Here's how the part is built. I have some questions about the finished solid (model axes, mm). A direction names the side the tool comes from. Coordinates: 2 decimals unless noted, no trailing zeros. Use a Markdown table: item, result. Add a question column.
Item 1: On a 3-axis mill with a long thin cutter (end or side, diameter ignored), from which of +Z, -Z, +X, -X, +Y, -Y can I reach the whole of each face in a straight line? I mean faces 5 (the flat face through (60, -156, 18.2)), 6 (the flat face through (43.6, -167, 1)), 7 (the flat face through (-43.6, -167, 1)). Say none if no direction works.
Item 2: Will these pins go through, and if not, where does the flat tip stop? pin 1 Ø2.5 at (y, z) = (-168, 2) entering from -X; pin 2 Ø4 at (y, z) = (-163, 25) entering from -X; pin 3 Ø8 at (x, y) = (6, -167) entering from +Z; pin 4 Ø1 at (x, z) = (28, 8) entering from -Y.
Item 3: If I drill on line 1 along Y through (x, z) = (26, 23); line 2 along X through (y, z) = (-155.25, 15.75); line 3 along Z through (x, y) = (-3.5, -165.5), over which ranges is the centre line in solid material (lowest first)? Write a range as from..to.
Item 4: If we mould it in two halves opening along Y, with no side actions, what happens to faces 1 (the flat face through (-53.8, -154, 17)), 2 (the cylindrical face through (-0.84, -150.65, 2)), 3 (the flat face through (-1, -155.949, 17)), 4 (the flat face through (-60, -156, 28.4))? For each: pulls with the +Y half, pulls with the -Y half, needs draft (parallel to the pull), parting line crosses it, or undercut.
```python
from build123d import *

# Parameters (mm, degrees)
EXTRUDE1_DEPTH     = 3
SKETCH3_W          = 134.4
SKETCH3_H          = 13.4
EXTRUDE2_DEPTH     = 7.4
SKETCH4_W          = 134.4
SKETCH4_H          = 13.4
SKETCH4_W_2        = 107.6
SKETCH4_H_2        = 4.4
EXTRUDE3_DEPTH     = 13
FILLET1_R          = 7
CUT_EXTRUDE1_DEPTH = 3
FILLET2_R          = 1.5
SKETCH7_R          = 2.5
EXTRUDE4_DEPTH     = 5
EXTRUDE4_TAPER     = 4
SKETCH8_R          = 2.6
CUT_EXTRUDE2_DEPTH = 5.2
CUT_EXTRUDE2_DRAFT = -3.8


with BuildPart() as part:
    # Sketch1 → Extrude1 (new body)
    with BuildSketch(Plane.XY):
        Polygon((-43.6, -161.948648405), (-43.6, -171.948648405), (43.6, -171.948648405), (43.6, -161.948648405), (67.2, -161.948648405), (67.2, -148.548648405), (-67.2, -148.548648405), (-67.2, -161.948648405), align=None)
    extrude(amount=EXTRUDE1_DEPTH)

    # Sketch3 → Extrude2 (add)
    with BuildSketch(Plane.XY.offset(3)):
        with Locations((0, -155.248648405)):
            Rectangle(SKETCH3_W, SKETCH3_H)
    extrude(amount=EXTRUDE2_DEPTH)

    # Sketch4 → Extrude3 (add)
    with BuildSketch(Plane.XY.offset(10.4)):
        with Locations((0, -155.248648405)):
            Rectangle(SKETCH4_W, SKETCH4_H)
        with Locations((0, -153.748648405)):
            Rectangle(SKETCH4_W_2, SKETCH4_H_2, mode=Mode.SUBTRACT)
    extrude(amount=EXTRUDE3_DEPTH)

    # Fillet1
    fillet1_edges = [part.edges().sort_by_distance(p)[0] for p in [
        (-67.2, -148.548648405, 11.7),
        (67.2, -148.548648405, 11.7),
        (-67.2, -155.248648405, 0),
        (0, -148.548648405, 0),
        (67.2, -155.248648405, 0),
    ]]
    fillet(fillet1_edges, radius=FILLET1_R)

    # Sketch6 → Cut-Extrude1 (cut)
    with BuildSketch(Plane.XZ.offset(161.948648405)):
        with BuildLine():
            Line((-55.3, 23.4), (-55.3, 18.9))
            ThreePointArc((-55.3, 18.9), (-53.249747468, 13.950252532), (-48.3, 11.9))
            Line((-48.3, 11.9), (48.3, 11.9))
            ThreePointArc((48.3, 11.9), (53.249747468, 13.950252532), (55.3, 18.9))
            Line((55.3, 18.9), (55.3, 23.4))
            Line((55.3, 23.4), (-55.3, 23.4))
        make_face()
    extrude(amount=-CUT_EXTRUDE1_DEPTH, mode=Mode.SUBTRACT)

    # Fillet2
    fillet2_edges = [part.edges().sort_by_distance(p)[0] for p in [
        (55.3, -158.948648405, 21.15),
        (53.249747468, -158.948648405, 13.950252532),
        (0, -158.948648405, 11.9),
        (-53.249747468, -158.948648405, 13.950252532),
        (-55.3, -158.948648405, 21.15),
        (-55.3, -161.948648405, 21.15),
        (-53.249747468, -161.948648405, 13.950252532),
        (55.3, -161.948648405, 21.15),
        (53.249747468, -161.948648405, 13.950252532),
        (0, -161.948648405, 11.9),
    ]]
    fillet(fillet2_edges, radius=FILLET2_R - 0.0001)  # a hair under: the kernel refuses the full size

    # Sketch7 → Extrude4 (add)
    with BuildSketch(Plane.XY.offset(23.4)):
        with Locations((-60.2, -155.548648405)):
            Circle(SKETCH7_R)
    extrude(amount=EXTRUDE4_DEPTH, taper=EXTRUDE4_TAPER)


with BuildPart() as cut_extrude2_tool:
    # Sketch8 → Cut-Extrude2 (with draft: the straight prism first)
    with BuildSketch(Plane.XY.offset(23.4)):
        with Locations((60.2, -155.548648405)):
            Circle(SKETCH8_R)
    extrude(amount=-CUT_EXTRUDE2_DEPTH)
    # Cut-Extrude2: the draft: its side faces are tilted about the plane it starts from
    cut_extrude2_sides = [cut_extrude2_tool.faces().sort_by_distance(p)[0] for p in [
        (57.6, -155.548648405, 20.8),
    ]]
    draft(cut_extrude2_sides, Plane.XY.offset(23.4), CUT_EXTRUDE2_DRAFT)


with BuildPart() as part_1:
    add(part.part)

    # Cut-Extrude2: cut by cut_extrude2_tool
    add(cut_extrude2_tool.part, mode=Mode.SUBTRACT)


solid = part_1.part
```
Ans:
| question | item | result |
|---|---|---|
| 1 | face 5 | +Z |
| 1 | face 6 | +Z, -Z, +X, -Y |
| 1 | face 7 | +Z, -Z, -X, -Y |
| 2 | pin 1 | stops at x = -43.6 |
| 2 | pin 2 | stops at x = -67.2 |
| 2 | pin 3 | stops at z = 3 |
| 2 | pin 4 | stops at y = -161.95 |
| 3 | line 1 | y = -158.95..-155.95, -151.55..-148.55 |
| 3 | line 2 | x = -67.19..-53.8, 53.8..67.19 |
| 3 | line 3 | z = 0..3 |
| 4 | face 1 | undercut |
| 4 | face 2 | pulls with the +Y half |
| 4 | face 3 | undercut |
| 4 | face 4 | needs draft |
